```python
from build123d import *

# Parameters (mm, degrees)
SKETCH001_R  = 4
PAD004_DEPTH = 31
PAD006_DEPTH = 4
SKETCH_R     = 4.1
PAD_DEPTH    = 80


with BuildPart() as rodhole02:
    # Sketch001 → Pad004 (new body)
    with BuildSketch(Plane.YZ.offset(15.5)):
        with Locations((-3.5, 70)):
            Circle(SKETCH001_R)
        with Locations((-3.5, 10)):
            Circle(SKETCH001_R)
    extrude(amount=-PAD004_DEPTH)


with BuildPart() as cutblock:
    # Sketch002 → Pad006 (new body)
    with BuildSketch(Plane.YZ.offset(-10)):
        Polygon((2.908588, 66.3), (2.908588, 73.7), (-3.5, 77.4), (-9.908588, 73.7), (-9.908588, 66.3), (-3.5, 62.6), align=None)
        Polygon((-3.5, 2.6), (2.908588, 6.3), (2.908588, 13.7), (-3.5, 17.4), (-9.908588, 13.7), (-9.908588, 6.3), align=None)
    extrude(amount=-PAD006_DEPTH)

    # Fusion: union RodHole02
    add(rodhole02.part)


with BuildPart() as cut:
    # Sketch → Pad (new body)
    with BuildSketch(Plane.XY):
        with BuildLine():
            Line((-13.000011, 5.000021), (-13.000011, -13))
            Line((-13.000011, -13), (13.000011, -13))
            Line((13.000011, -13), (13.000011, 13))
            Line((13.000011, 13), (-5.00001, 13))
            ThreePointArc((-5.00001, 13), (-10.656858, 10.656862), (-13.000011, 5.000021))
        make_face()
        with Locations((-5.000011, 5)):
            Circle(SKETCH_R, mode=Mode.SUBTRACT)
    extrude(amount=PAD_DEPTH)

    # Cut: cut CutBlock
    add(cutblock.part, mode=Mode.SUBTRACT)


solid = cut.part
```
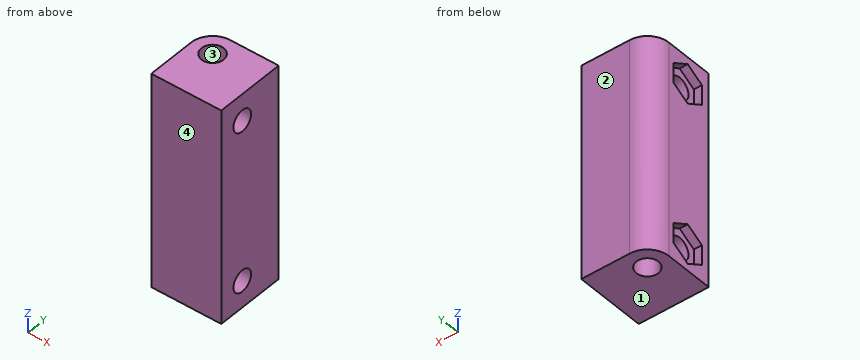
Check sheet for the modelled part. Datum: model origin and axes. Units: mm. Face numbers are marked on the shaded views. Coordinates: 2 decimals unless noted, no trailing zeros. Order: outer loops, then holes, each group sorted by start corner. A loop starts at its lowest first (then second) coordinate and runs counter-clockwise, first axis right, second up. Notation, with made-up numbers: (1.25, 64) -> (36.25, 64) arc R24 cw to (36.25, 88) -> close; hole circle Ø2 at (15.5, -3.5). An arc over 180 degrees is marked (long way). Write each question's results on one line, items separated by ' | '. Start each with the question number.
1) Depth check by flat-ended pin: pin 1 (6 mm diameter, centred on y = 9, z = 11.5, fed in from -X); pin 2 (0.9 mm diameter, centred on x = -11.5, z = 10, fed in from +Y); pin 3 (1.5 mm diameter, centred on x = -11.5, z = 71, fed in from +Y). Enter the tip coordinate at first touch or a pass-through.
2) Section check C-C (x = 3). Enter the section's corners in (y, z), and give its area (3 significant figures).
3) Section check B-B (y = -5.25). Enter the section's corners in (x, z).
4) Material ranges on line 1 along Z through (x, y) = (3.25, -3.5); line 2 along Y through (x, z) = (-3, 69.5); line 3 along Z through (x, y) = (-2, -6), recorded low to high.
5) Section check A-A (z = 70). Enter the section's corners in (x, y).
6) Draft check along Y on the marked faces 1, 2, 3 and 4. Enter one of: pulls with the +Y half, pulls with the -Y half, needs draft (parallel to the pull), parting line crosses it, or undercut.
7) Section check D-D (y = 7). Enter the section's corners in (x, z), and give its area (3 significant figures).
Checked values:
1) pin 1: x = -12.94 | pin 2: y = 10.23 | pin 3: y = 10.56
2) outline: (-13, 0) -> (13, 0) -> (13, 80) -> (-13, 80) -> close; hole circle Ø8 at (-3.5, 10); hole circle Ø8 at (-3.5, 70) | area: 1,980 mm²
3) outline: (-13, 0) -> (13, 0) -> (13, 6.4) -> (-10, 6.4) -> (-10, 3.61) -> (-13, 3.61) -> close; (-13, 16.39) -> (-10, 16.39) -> (-10, 13.6) -> (13, 13.6) -> (13, 66.4) -> (-10, 66.4) -> (-10, 63.61) -> (-13, 63.61) -> close; (-13, 76.39) -> (-10, 76.39) -> (-10, 73.6) -> (13, 73.6) -> (13, 80) -> (-13, 80) -> close
4) line 1: 0 to 6, 14 to 66, 74 to 80 | line 2: -13 to -7.47, 0.47 to 1.42, 8.58 to 13 | line 3: 0 to 6.88, 13.12 to 66.88, 73.12 to 80
5) outline: (-13, -13) -> (13, -13) -> (13, -7.5) -> (-10, -7.5) -> (-10, -9.91) -> (-13, -9.91) -> close; (-13, 2.91) -> (-10, 2.91) -> (-10, 0.5) -> (13, 0.5) -> (13, 13) -> (-5, 13) arc R8 ccw to (-13, 5) -> close; hole circle Ø8.2 at (-5, 5)
6) face 1: needs draft | face 2: pulls with the +Y half | face 3: undercut | face 4: pulls with the -Y half
7) outline: (-12.75, 0) -> (-8.58, 0) -> (-8.58, 80) -> (-12.75, 80) -> close; (-1.42, 0) -> (13, 0) -> (13, 80) -> (-1.42, 80) -> close | area: 1,490 mm²
